Work out the finished part from the listing and answer in its coordinate system (mm). A direction names the side the tool comes from. Give positions to 0.01 mm unless a question says otherwise; leave off trailing zeros. Loops run counter-clockwise (first coordinate to the right, second up) from the corner with the lowest first, then second, coordinate; pieces in that order, holes last. Notation, with made-up numbers: (-18.5, -30.5) - (18.5, -30.5) arc R22 cw to (18.5, -16.5) - close; hole circle Ø6 at (-22, -30.75). An arc over 180 degrees is marked (long way). One line per question, with ' | ' between items. Start each with the question number.
1. Find the intervals of material crossed by line 1 (X direction, y = 0, z = 20); line 2 (Y direction, x = 0, z = 45.5), in increasing order.
2. Which of the six approach directions +Z, -Z, +X, -X, +Y, -Y give full straight-line access (tool end or side, diameter ignored) to faces 1 (the face through (-10, 0, 45)), 2 (the face through (-2.38, -10.74, 22.18))?
3. Section D-D (z = 8) is taken. Determine the outline of the cut face in (x, y), plus the area to 3 significant figures.
4. For a pull along X with two mould halves and no side action, classify faces 3 (the face through (4.38, -8.43, 72.11)), 4 (the face through (6.235, -2.585, 49.3)), 5 (the face through (4, -6, 100)) as released by +X, released by -X, zero draft, split by the parting line, or undercut.
5. Section A-A (x = 0) is taken. Determine the outline of the cut face in (y, z).
6. Section B-B (y = -4) is taken. Determine the outline of the cut face in (x, z), plus the area to 3 significant figures.
7. Each of these flat-tipped pins is pushed along its axis until it touches: pin 1 (8 mm diameter, centred on y = 8.5, z = 60.5, fed in from -X); pin 2 (8 mm diameter, centred on y = 6.5, z = 21, fed in from -X); pin 3 (1 mm diameter, centred on x = 1.5, z = 17.5, fed in from +Y); pin 4 (11 mm diameter, centred on x = 0, y = 0, fed in from -Z). Where does it stop, or does it pass through?
8. Section C-C (x = -7.75) is taken. Determine the outline of the cut face in (y, z), plus the area to 3 significant figures.
from build123d import *

# Parameters (mm, degrees)
F0_R     = 11
F0_R_2   = 6.75
F1_DEPTH = 45
F2_R     = 9.5
F2_R_2   = 6.75
F3_DEPTH = 55
F5_DEPTH = 12.0000001


with BuildPart() as f1:
    # F0 (on Top) → F1 (new body)
    with BuildSketch(Plane.XY):
        Circle(F0_R)
        Circle(F0_R_2, mode=Mode.SUBTRACT)
    extrude(amount=F1_DEPTH)

    # F2 (on face) → F3 (join)
    with BuildSketch(Plane.XY.offset(45)):
        Circle(F2_R)
        Circle(F2_R_2, mode=Mode.SUBTRACT)
    extrude(amount=F3_DEPTH)

    # F4 (on Right) → F5 (cut, up to face)
    with BuildSketch(Plane.YZ):
        with BuildLine():
            ThreePointArc((0, 3.25), (1.2374368671, 3.7625631329), (1.75, 5))
            ThreePointArc((1.75, 5), (-1.2374368671, 6.2374368671), (0, 3.25))
        make_face()
    extrude(amount=-F5_DEPTH, mode=Mode.SUBTRACT)


solid = f1.part
Conclusion:
1) line 1: -11 to -6.75, 6.75 to 11 | line 2: -9.5 to -6.75, 6.75 to 9.5
2) face 1: +Z | face 2: +Z, -Z
3) outline: circle Ø22 at (0, 0); hole circle Ø13.5 at (0, 0) | area: 237 mm²
4) face 3: split by the parting line | face 4: undercut | face 5: zero draft
5) outline: (-11, 0) - (-6.75, 0) - (-6.75, 100) - (-9.5, 100) - (-9.5, 45) - (-11, 45) - close; (6.75, 0) - (11, 0) - (11, 45) - (9.5, 45) - (9.5, 100) - (6.75, 100) - close
6) outline: (-10.25, 0) - (-5.44, 0) - (-5.44, 100) - (-8.62, 100) - (-8.62, 45) - (-10.25, 45) - close; (5.44, 0) - (10.25, 0) - (10.25, 45) - (8.62, 45) - (8.62, 100) - (5.44, 100) - close | area: 783 mm²
7) pin 1: x = -8.37 | pin 2: x = -10.71 | pin 3: y = 10.95 | pin 4: through
8) outline: (-7.81, 0) - (7.81, 0) - (7.81, 45) - (5.49, 45) - (5.49, 100) - (-5.49, 100) - (-5.49, 45) - (-7.81, 45) - close; hole circle Ø3.5 at (0, 5) | area: 1,300 mm²
